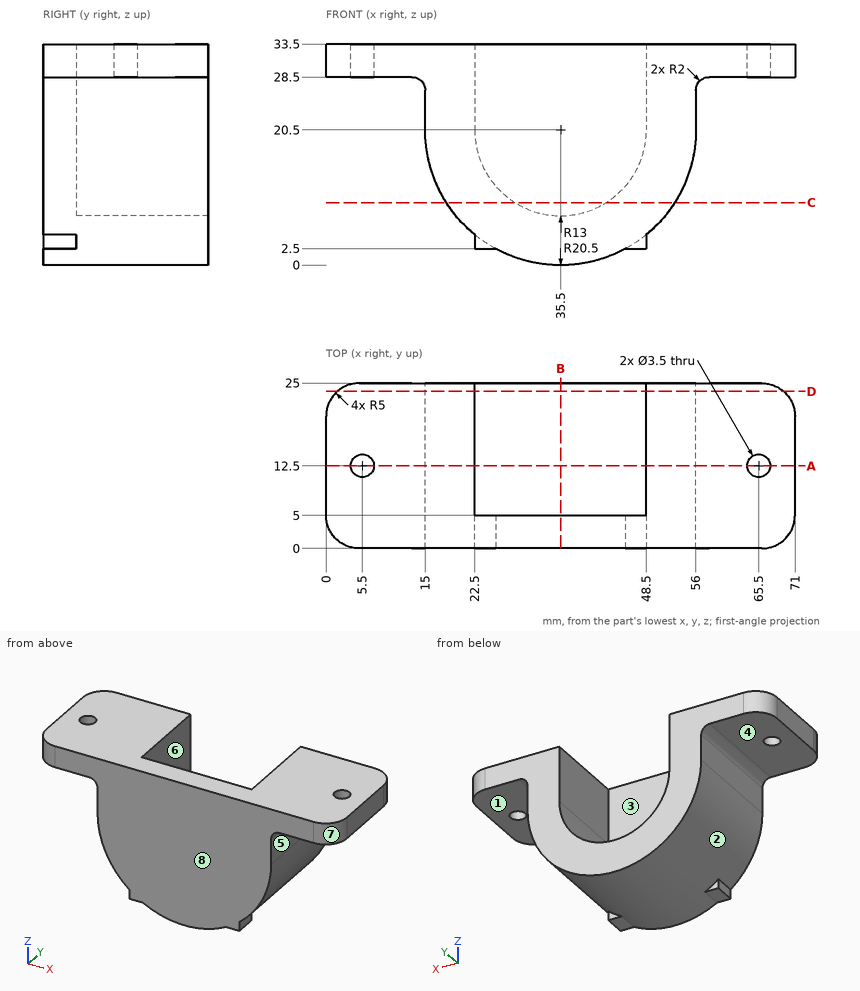
Study the drawing (mm; zero at the part's minimum x, y, z) and answer. A direction names the side the tool comes from. Round coordinates to 2 decimals unless told otherwise and drop trailing zeros. Order: outer loops, then holes, each group sorted by start corner. A loop starts at its lowest first (then second) coordinate and runs counter-clockwise, first axis right, second up. Notation, with made-up numbers: (65, 86.25) - (110, 86.25) arc R21 ccw to (110, 116.25) - close; hole circle Ø11 at (-29, 6.25). An arc over 180 degrees is marked (long way). Use one line per item in the form item = value. Start each with the question number.
(1) The part is cut by section B-B (x = 35.5). Give the vertices of the cut face in (y, z), then the cut area to 4 significant figures.
(2) Determine the mould class of the marked faces 1, 2 and 3 for opening direction X: +X half, -X half, draft (parallel to the pull), parting line (faces both ways), or undercut.
(3) For the marked faces 4, 5, 6, 7 and 8, determine the directions among +Z, -Z, +X, -X, +Y, -Y from which every point of the face is accessible in a straight line to the end or side of a thin tool.
(4) The part is cut by section C-C (z = 9.5). Give the vertices of the cut face in (x, y).
(5) The part is cut by section D-D (y = 23.75). Give the vertices of the cut face in (x, z), then the cut area to 3 significant figures.
(6) Find the intervals of material crossed by line 1 along Y through (x, z) = (5.5, 31.75); line 2 along X through (y, z) = (19, 24.5); line 3 along Z through (x, y) = (66.5, 1.5), in increasing order. Write a range as from..to.
(7) Flat-ended cylindrical pins translate along their axes: pin 1 Ø4 at (x, y) = (45.5, 17) entering from +Z; pin 2 Ø2.5 at (x, z) = (24, 3.5) entering from +Y; pin 3 Ø10.5 at (x, y) = (61.5, 9) entering from -Z; pin 4 Ø2.5 at (x, y) = (47.5, 3) entering from -Z. Find the tip coordinate at first contact, or state that the pin passes through.
(8) The part is cut by section A-A (y = 12.5). Give the vertices of the cut face in (x, z), then the cut area to 3 significant figures.
Checked values:
q1.outline = (0, 0) - (25, 0) - (25, 7.5) - (5, 7.5) - (5, 33.5) - (0, 33.5) - close
q1.area = 317.5 mm^2
q2.face_1 = draft
q2.face_2 = parting line
q2.face_3 = undercut
q3.face_4 = -Z, -X, +Y, -Y
q3.face_5 = -Z, +X, +Y, -Y
q3.face_6 = +Z, +Y
q3.face_7 = +Z, -Z, +X, -Y
q3.face_8 = +Z, -Z, +X, -X, -Y
q4.outline = (18.2, 0) - (52.8, 0) - (52.8, 25) - (42.43, 25) - (42.43, 5) - (28.57, 5) - (28.57, 25) - (18.2, 25) - close
q5.outline = (1.69, 28.5) - (13, 28.5) arc R2 cw to (15, 26.5) - (15, 20.5) arc R20.5 ccw to (56, 20.5) - (56, 26.5) arc R2 cw to (58, 28.5) - (69.31, 28.5) - (69.31, 33.5) - (48.5, 33.5) - (48.5, 20.5) arc R13 cw to (22.5, 20.5) - (22.5, 33.5) - (1.69, 33.5) - close
q5.area = 724 mm^2
q6.line_1 = 0..10.75, 14.25..25
q6.line_2 = 15..22.5, 48.5..56
q6.line_3 = 28.5..33.5
q7.pin_1 = 15.5
q7.pin_2 = 25
q7.pin_3 = 27.47
q7.pin_4 = 2.5
q8.outline = (0, 28.5) - (3.75, 28.5) - (3.75, 33.5) - (0, 33.5) - close; (7.25, 28.5) - (13, 28.5) arc R2 cw to (15, 26.5) - (15, 20.5) arc R20.5 ccw to (56, 20.5) - (56, 26.5) arc R2 cw to (58, 28.5) - (63.75, 28.5) - (63.75, 33.5) - (48.5, 33.5) - (48.5, 20.5) arc R13 cw to (22.5, 20.5) - (22.5, 33.5) - (7.25, 33.5) - close; (67.25, 28.5) - (71, 28.5) - (71, 33.5) - (67.25, 33.5) - close
q8.area = 706 mm^2
